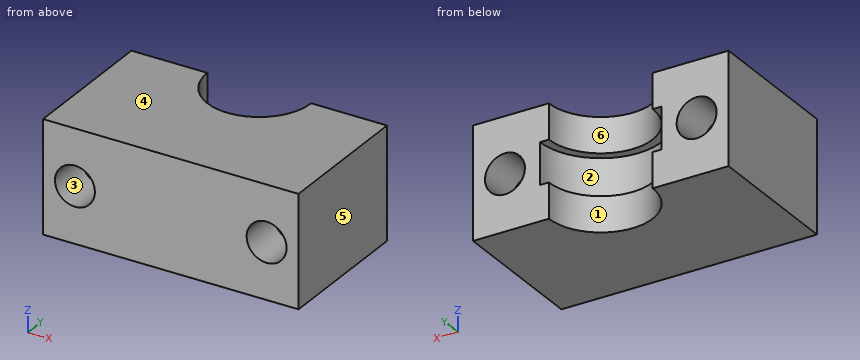
from build123d import *

# Parameters (mm, degrees)
SKETCH_1_W               = 32
SKETCH_1_H               = 14
EXTRUDE_1_DEPTH          = 18
SKETCH_3_R               = 7.6
CUT_EXTRUDE_1_DEPTH      = 2.6
CUT_EXTRUDE_2_DEPTH      = 26.079872408
CUT_EXTRUDE_2_DEPTH_BACK = 26.079872408
SKETCH_4_R               = 6.5
SKETCH_5_R               = 2.5
CUT_EXTRUDE_3_DEPTH      = 5.5


with BuildPart() as part:
    # 草圖1 → 填料-伸長1 (new body)
    with BuildSketch(Plane(origin=(0, 0, 0), x_dir=(1, 0, 0), z_dir=(0, 1, 0))):
        Rectangle(SKETCH_1_W, SKETCH_1_H)
    extrude(amount=EXTRUDE_1_DEPTH)

    # 草圖3 → 除料-伸長1 (cut, symmetric)
    with BuildSketch(Plane.XY):
        with Locations((0, 18)):
            Circle(SKETCH_3_R)
    extrude(amount=CUT_EXTRUDE_1_DEPTH, both=True, mode=Mode.SUBTRACT)

    # 草圖4 → 除料-伸長2 (cut, two sides: drawn at the far end of the back side and taken through both)
    with BuildSketch(Plane.XY.offset(-CUT_EXTRUDE_2_DEPTH_BACK)):
        with Locations((0, 18)):
            Circle(SKETCH_4_R)
    extrude(amount=CUT_EXTRUDE_2_DEPTH + CUT_EXTRUDE_2_DEPTH_BACK, mode=Mode.SUBTRACT)

    # 草圖5 → 除料-伸長3 (cut)
    with BuildSketch(Plane(origin=(0, 18, 0), x_dir=(1, 0, 0), z_dir=(0, 1, 0))):
        with Locations(Location((-12, 0, 0), (0, 0, 270))):
            Circle(SKETCH_5_R)
        with Locations(Location((12, 0, 0), (0, 0, 90))):
            Circle(SKETCH_5_R)
    cut_extrude_3 = extrude(amount=-CUT_EXTRUDE_3_DEPTH, mode=Mode.SUBTRACT)

    # Mirror1: 除料-伸長3 across plane
    add(cut_extrude_3.mirror(Plane.ZX.offset(9)), mode=Mode.SUBTRACT)


solid = part.part
Design review of the part built by this model. Coordinates are the model's own, in mm. Face numbers are marked on the shaded views. A direction names the side the tool comes from. Coordinates: 2 decimals unless noted, no trailing zeros. Write each loop counter-clockwise with the first axis right and the second up, starting at its lowest first coordinate (ties: lowest second). Pieces come first, ordered by that corner, then holes. Notation, with made-up numbers: (-23, 18) - (24, 18) arc R19 cw to (24, 46) - close; hole circle Ø7 at (61.5, 1.25). An arc over 180 degrees is marked (long way). Use one line per item in the form item = value.
Q1. Consider section A-A (z = 0). Write out the cut boundary in (x, y), plus the area to 3 significant figures.
Taken from the geometry:
outline = (-16, 0) - (-14.5, 0) - (-14.5, 5.5) - (-9.5, 5.5) - (-9.5, 0) - (9.5, 0) - (9.5, 5.5) - (14.5, 5.5) - (14.5, 0) - (16, 0) - (16, 18) - (14.5, 18) - (14.5, 12.5) - (9.5, 12.5) - (9.5, 18) - (7.6, 18) arc R7.6 cw to (-7.6, 18) - (-9.5, 18) - (-9.5, 12.5) - (-14.5, 12.5) - (-14.5, 18) - (-16, 18) - close
area = 375 mm^2
Q2. Consider section C-C (y = 1). Write out the cut boundary in (x, z), plus the area to 3 significant figures.
Taken from the geometry:
outline = (-16, -7) - (16, -7) - (16, 7) - (-16, 7) - close; hole circle Ø5 at (-12, 0); hole circle Ø5 at (12, 0)
area = 409 mm^2
Q3. Consider section D-D (x = 0). Write out the cut boundary in (y, z), plus the area to 3 significant figures.
Taken from the geometry:
outline = (0, -7) - (11.5, -7) - (11.5, -2.6) - (10.4, -2.6) - (10.4, 2.6) - (11.5, 2.6) - (11.5, 7) - (0, 7) - close
area = 155 mm^2
Q4. Insertion check: pin 1 Ø4.5 at (x, z) = (-12, 0) entering from +Y; pin 2 Ø1.5 at (x, z) = (1, -0.5) entering from +Y; pin 3 Ø4 at (x, z) = (4, 0) entering from +Y. Each pin has a flat end and moves straight along its axis. Give the tip position at first contact, or say it passes through.
Taken from the geometry:
pin_1 = 12.5
pin_2 = 10.6
pin_3 = 13.34
Q5. For probe 1 along X at (y, z) = (1.9, 0); probe 2 along X at (y, z) = (16, 0); probe 3 along Z at (x, y) = (12, 3.55), list the stretches that pass through material, from the lowest coordinate up.
Taken from the geometry:
probe_1 = -16 to -14.5, -9.5 to 9.5, 14.5 to 16
probe_2 = -16 to -14.5, -9.5 to -7.33, 7.33 to 9.5, 14.5 to 16
probe_3 = -7 to -2.5, 2.5 to 7
Q6. The part is to be moulded in two halves that separate along X. For the marked faces 4, 5 and 6, say which applies: +X half, -X half, draft (parallel to the pull), parting line (faces both ways), or undercut.
Taken from the geometry:
face_4 = draft
face_5 = +X half
face_6 = undercut
Q7. Consider section B-B (x = 12). Write out the cut boundary in (y, z).
Taken from the geometry:
outline = (0, -7) - (18, -7) - (18, -2.5) - (12.5, -2.5) - (12.5, 2.5) - (18, 2.5) - (18, 7) - (0, 7) - (0, 2.5) - (5.5, 2.5) - (5.5, -2.5) - (0, -2.5) - close
Q8. Machinability: for the marked faces 1, 2 and 3, which of the approach directions +Z, -Z, +X, -X, +Y, -Y give a long, thin tool a straight path to every point of the face, cutting with its end or side? Answer none if there is none.
Taken from the geometry:
face_1 = +Z, -Z, +Y
face_2 = +Y
face_3 = -Y
